```python
from build123d import *

# Parameters (mm, degrees)
SKETCH1_W                  = 177.8
SKETCH1_H                  = 25.4
BOSS_EXTRUDE1_DEPTH        = 9.525
F_1_2_0_5_DIAMETER_HOLE1_D = 12.7
CUT_EXTRUDE1_DEPTH         = 180.857514786


with BuildPart() as part:
    # Sketch1 → Boss-Extrude1 (new body)
    with BuildSketch(Plane.XY):
        with Locations((88.9, 12.7)):
            Rectangle(SKETCH1_W, SKETCH1_H)
    extrude(amount=BOSS_EXTRUDE1_DEPTH)

    # 1/2 (0.5) Diameter Hole1 (through all)
    with Locations(Plane.XY.offset(9.525)):
        with Locations((12.7, 12.7), (147.32, 12.7)):
            Hole(F_1_2_0_5_DIAMETER_HOLE1_D / 2)

    # Sketch5 → Cut-Extrude1 (cut, through all)
    with BuildSketch(Plane.XY.offset(9.525)):
        Polygon((13.208, 25.4), (0, 21.419090106), (0, 25.4), align=None)
    extrude(amount=-CUT_EXTRUDE1_DEPTH, mode=Mode.SUBTRACT)


solid = part.part
```
Geometry: final body of the model. Coordinates: model frame, mm. Round coordinates to 2 decimals unless told otherwise and drop trailing zeros. Order: outer loops, then holes, each group sorted by start corner. A loop starts at its lowest first (then second) coordinate and runs counter-clockwise, first axis right, second up. Notation, with made-up numbers: M -19,-14 L 28,-14 A26 cw 28,20 Z; hole C 52,39 d1. An arc over 180 degrees is marked long. Use one line per item in the form item = value. Start each with the question number.
Q1. Mould query, pull axis X, two halves, no side actions, for faces 1 (the face through (177.8, 13, 5)), 2 (the face through (94, 25.4, 5)), 3 (the face through (141.263, 14.607, 4.696)). Classes: +X half, -X half, draft (parallel to the pull), parting line (faces both ways), or undercut.
Q2. Cut plane B-B (y = 12.7). Return loops of the section in (x, z) (3 decimals), and give its area (3 significant figures).
Q3. Cut plane A-A (x = 147.32). Return loops of the section in (y, z) (3 decimals), and give its area (3 significant figures).
Q4. Cut plane C-C (z = 5.5). Return loops of the section in (x, y).
Q5. Material intervals for line 1 (Y direction, x = 147.32, z = 2.75); line 2 (X direction, y = 7, z = 7.5); line 3 (X direction, y = 18.5, z = 2.5), sorted ascending. Write a range as [from, to].
Q6. Pin query (flat end, axial travel): pin 1 Ø10 at (x, y) = (147.32, 12.7) entering from +Z. Return the tip coordinate at first contact, or that it passes through.
Geometry results:
q1.face_1 = +X half
q1.face_2 = draft
q1.face_3 = undercut
q2.outline = M 0,0 L 6.35,0 L 6.35,9.525 L 0,9.525 Z; M 19.05,0 L 140.97,0 L 140.97,9.525 L 19.05,9.525 Z; M 153.67,0 L 177.8,0 L 177.8,9.525 L 153.67,9.525 Z
q2.area = 1,450 mm^2
q3.outline = M 0,0 L 6.35,0 L 6.35,9.525 L 0,9.525 Z; M 19.05,0 L 25.4,0 L 25.4,9.525 L 19.05,9.525 Z
q3.area = 121 mm^2
q4.outline = M 0,0 L 177.8,0 L 177.8,25.4 L 13.21,25.4 L 0,21.42 Z; hole C 12.7,12.7 d12.7; hole C 147.32,12.7 d12.7
q5.line_1 = [0, 6.35], [19.05, 25.4]
q5.line_2 = [0, 9.9], [15.5, 144.52], [150.12, 177.8]
q5.line_3 = [0, 10.11], [15.29, 144.73], [149.91, 177.8]
q6.pin_1 = through
